from build123d import *

# Parameters (mm, degrees)
F0_R     = 1.35
F1_DEPTH = 6


with BuildPart() as f1:
    # F0 (on Front) → F1 (new body)
    with BuildSketch(Plane.XZ):
        with BuildLine():
            ThreePointArc((0, 25.2), (-21.1, 4.1), (0, -17))
            Line((0, -17), (13.8, -17))
            Line((13.8, -17), (13.8, -10.8))
            Line((13.8, -10.8), (8, -10.8))
            Line((8, -10.8), (8, -5))
            Line((8, -5), (13.8, -5))
            Line((13.8, -5), (13.8, 1.2))
            Line((13.8, 1.2), (8, 1.2))
            Line((8, 1.2), (8, 7))
            Line((8, 7), (13.8, 7))
            Line((13.8, 7), (13.8, 13.2))
            Line((13.8, 13.2), (8, 13.2))
            Line((8, 13.2), (8, 19))
            Line((8, 19), (13.8, 19))
            Line((13.8, 19), (13.8, 25.2))
            Line((13.8, 25.2), (0, 25.2))
        make_face()
        Circle(F0_R, mode=Mode.SUBTRACT)
        with Locations((-7, 12.124356)):
            Circle(F0_R, mode=Mode.SUBTRACT)
    extrude(amount=F1_DEPTH)


solid = f1.part
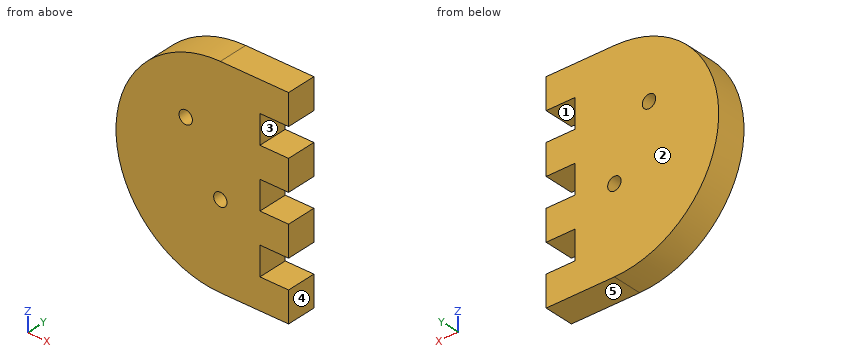
Source: CAD feature listing. Evaluate the final solid. Frame: model axes, mm. Face numbers are marked on the shaded views. A direction names the side the tool comes from. Coordinates: 2 decimals unless noted, no trailing zeros. Loops run counter-clockwise (first coordinate to the right, second up) from the corner with the lowest first, then second, coordinate; pieces in that order, holes last. Notation, with made-up numbers: M -40,-8.5 L -15,-8.5 A15 ccw -15,-2.5 Z; hole C -16.75,-28 d7. An arc over 180 degrees is marked long. Answer in a Markdown table with one row per item.
Q1. Section D-D on z = 21. Return the cut outline in (x, y).
Answers below:
| item | result |
|---|---|
| outline | M -12.63,-6 L 13.8,-6 L 13.8,0 L -12.63,0 Z |
Q2. Ray query, probe 1 along Z at (x, y) = (0, -1.6); probe 2 along X at (y, z) = (-4.6, 0.5); probe 3 along Z at (x, y) = (-7, -2.35). Return the intervals inside material, ascending. Write a range as from..to.
Answers below:
| item | result |
|---|---|
| probe 1 | z = -17..-1.35, 1.35..25.2 |
| probe 2 | x = -20.79..-1.25, 1.25..13.8 |
| probe 3 | z = -15.81..10.77, 13.47..24.01 |
Q3. Draft query along Z for the marked faces 3, 4 and 5. Return one class per face: pulls with the +Z half, pulls with the -Z half, needs draft (parallel to the pull), parting line crosses it, or undercut.
Answers below:
| item | result |
|---|---|
| face 3 | undercut |
| face 4 | needs draft |
| face 5 | pulls with the -Z half |
Q4. Section A-A on y = -2.35. Return the cut outline in (x, z).
Answers below:
| item | result |
|---|---|
| outline | M 0,-17 L 13.8,-17 L 13.8,-10.8 L 8,-10.8 L 8,-5 L 13.8,-5 L 13.8,1.2 L 8,1.2 L 8,7 L 13.8,7 L 13.8,13.2 L 8,13.2 L 8,19 L 13.8,19 L 13.8,25.2 L 0,25.2 A21.1 ccw Z; hole C -7,12.12 d2.7; hole C 0,0 d2.7 |
Q5. Section B-B on x = -7. Return the cut outline in (y, z).
Answers below:
| item | result |
|---|---|
| outline | M -6,-15.81 L 0,-15.81 L 0,10.77 L -6,10.77 Z; M -6,13.47 L 0,13.47 L 0,24.01 L -6,24.01 Z |
Q6. Section C-C on z = 0. Return the cut outline in (x, y).
Answers below:
| item | result |
|---|---|
| outline | M -20.7,-6 L -1.35,-6 L -1.35,0 L -20.7,0 Z; M 1.35,-6 L 13.8,-6 L 13.8,0 L 1.35,0 Z |
Q7. Set-up query: the marked faces 1 and 2. Return all of +Z, -Z, +X, -X, +Y, -Y with unobstructed straight access to the full face (end or side cutting, diameter ignored); none if empty.
Answers below:
| item | result |
|---|---|
| face 1 | +X, +Y, -Y |
| face 2 | +Z, -Z, +X, -X, +Y |
Q8. First-contact query: pin 1 (3 mm diameter, centred on y = -4, z = 5.5, fed in from -X); pin 2 (2 mm diameter, centred on y = -2, z = -9.5, fed in from +X); pin 3 (2 mm diameter, centred on y = -2.5, z = -2, fed in from -X). Flat tips, straight axial feed; report the tip coordinate or a pass-through.
Answers below:
| item | result |
|---|---|
| pin 1 | stops at x = -21.1 |
| pin 2 | stops at x = 8 |
| pin 3 | stops at x = -20.47 |
